CAD build for the part. Positions are in the model's coordinates, mm. Round coordinates to 2 decimals unless told otherwise and drop trailing zeros. Order: outer loops, then holes, each group sorted by start corner. A loop starts at its lowest first (then second) coordinate and runs counter-clockwise, first axis right, second up. Notation, with made-up numbers: M 4.25,-32.75 L 32.25,-32.75 A9 ccw 32.25,-22.75 Z; hole C 13.25,37.25 d4. An arc over 180 degrees is marked long. Put each result on its own line as item: value.
```python
from build123d import *

# Parameters (mm, degrees)
SKETCH1_R           = 2.3495
BOSS_EXTRUDE2_DEPTH = 1.6002


with BuildPart() as part:
    # Sketch1 → Boss-Extrude2 (new body)
    with BuildSketch(Plane.XY):
        with BuildLine():
            Line((45.72, 5.08), (45.72, 172.72))
            ThreePointArc((45.72, 172.72), (40.512358569, 185.292358569), (27.94, 190.5))
            Line((27.94, 190.5), (17.78, 190.5))
            ThreePointArc((17.78, 190.5), (5.207641431, 185.292358569), (0, 172.72))
            Line((0, 172.72), (0, 4.761637225))
            ThreePointArc((0, 4.761637225), (1.592291129, 1.377049629), (5.070014314, 0))
            Line((5.070014314, 0), (33.655, 0))
            Line((33.655, 0), (40.64, 0))
            ThreePointArc((40.64, 0), (44.232102448, 1.487897552), (45.72, 5.08))
        make_face()
        with Locations((33.655, 24.13)):
            Circle(SKETCH1_R, mode=Mode.SUBTRACT)
        with Locations((33.655, 64.77)):
            Circle(SKETCH1_R, mode=Mode.SUBTRACT)
        with Locations((33.655, 113.03)):
            Circle(SKETCH1_R, mode=Mode.SUBTRACT)
        with Locations((33.655, 153.67)):
            Circle(SKETCH1_R, mode=Mode.SUBTRACT)
        with Locations((13.208, 7.15102725)):
            Circle(SKETCH1_R, mode=Mode.SUBTRACT)
        with Locations((13.208, 67.603137295)):
            Circle(SKETCH1_R, mode=Mode.SUBTRACT)
    extrude(amount=BOSS_EXTRUDE2_DEPTH)


solid = part.part
```
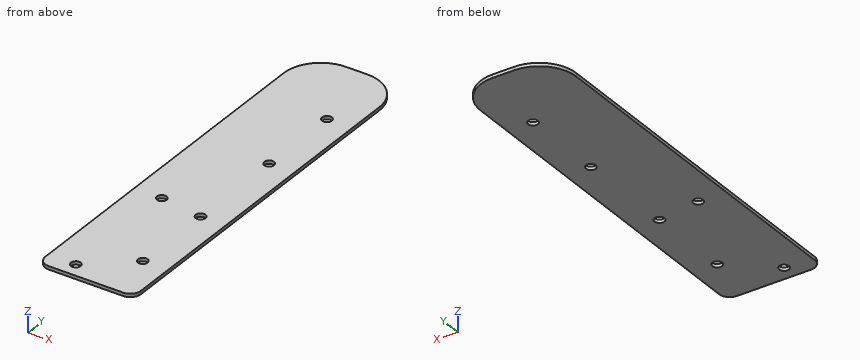
Item 1: Band-saw the part on A-A on y = 24.13. Give the cut face in (x, z), and give its area (3 significant figures).
Answers below:
outline: M 0,0 L 31.31,0 L 31.31,1.6 L 0,1.6 Z; M 36,0 L 45.72,0 L 45.72,1.6 L 36,1.6 Z
area: 65.6 mm²
Item 2: Probe line 1 along X through (y, z) = (66, 1.4); line 2 along Y through (x, z) = (15, 1.55); line 3 along Y through (x, z) = (35, 1.25). List the from-to ranges inside material, lowest first. Write a range as [from, to].
Answers below:
line 1: [0, 11.49], [14.93, 31.65], [35.66, 45.72]
line 2: [0, 5.63], [8.67, 66.08], [69.12, 190.28]
line 3: [0, 22.2], [26.06, 62.84], [66.7, 111.1], [114.96, 151.74], [155.6, 189.04]
Item 3: Band-saw the part on C-C on x = 38. Give the cut face in (y, z).
Answers below:
outline: M 0,0 L 187.38,0 L 187.38,1.6 L 0,1.6 Z
Item 4: Pin check, flat tip, straight feed: P1, Ø3, axis at x = 13.21, y = 67.6, coming from the +Z side. Stop position of the tip, or through.
Answers below:
P1: through
Item 5: Band-saw the part on B-B on z = 1.05. Give the cut face in (x, y) (1 decimal).
Answers below:
outline: M 0,4.8 A5.1 ccw 5.1,0 L 40.6,0 A5.1 ccw 45.7,5.1 L 45.7,172.7 A17.8 ccw 27.9,190.5 L 17.8,190.5 A17.8 ccw 0,172.7 Z; hole C 13.2,7.2 d4.7; hole C 13.2,67.6 d4.7; hole C 33.7,24.1 d4.7; hole C 33.7,64.8 d4.7; hole C 33.7,113 d4.7; hole C 33.7,153.7 d4.7
Item 6: Band-saw the part on D-D on x = 3.5. Give the cut face in (y, z).
Answers below:
outline: M 0.25,0 L 183.31,0 L 183.31,1.6 L 0.25,1.6 Z
